The model under review builds one solid part; all positions refer to its coordinate system, in mm. A direction names the side the tool comes from. Round coordinates to 2 decimals unless told otherwise and drop trailing zeros. Write each loop counter-clockwise with the first axis right and the second up, starting at its lowest first coordinate (ties: lowest second). Pieces come first, ordered by that corner, then holes.
Item 1: Draft analysis for pull direction X (two halves, no side actions). For faces 1 (the face through (5.86, 20.83, 6.6)), 2 (the face through (236.99, 31.15, 0.49)), 3 (the face through (118.226, 4.257, 1.521)), 4 (the face through (118, 17, 0)), state which applies: +X half, -X half, draft (parallel to the pull), parting line (faces both ways), or undercut.
Item 2: Machinability: for faces 5 (the face through (118, 8, 4)), 6 (the face through (118, 17, 4)), 7 (the face through (5.86, 16.93, 3.17)), 8 (the face through (234.14, 13.17, 6.72)), 9 (the face through (118, 26, 4)), which of the approach directions +Z, -Z, +X, -X, +Y, -Y give a long, thin tool a straight path to every point of the face, cutting with its end or side? Answer none if there is none.
Item 3: To check wall thickness, follow L1, parallel to Y at x = 26, z = 7; L2, parallel to X at y = 27, z = 2.75; L3, parallel to Y at x = 120, z = 1.7. State the ranges of each line that lie inside material, in increasing order.
Item 4: Clearance check with flat-ended pins moving along their axes: pin 1 Ø3.5 at (x, y) = (124, 6.5) entering from +Z; pin 2 Ø2 at (y, z) = (9.5, 1.5) entering from +X; pin 3 Ø3.5 at (x, z) = (101.5, 9) entering from -Y; pin 4 Ø3 at (x, z) = (70, 8.5) entering from +Y. State where each tip first meets the part, or that it passes through.
Item 5: Add section A-A (z = 8.25). Give the boundary of the cut face in (x, y), plus the area to 3 significant figures.
Item 6: Add section B-B (x = 60). Give the boundary of the cut face in (y, z).
```python
from build123d import *

# Parameters (mm, degrees)
PAD_DEPTH       = 240
FILLET_R        = 10
FILLET001_R     = 3
CHAMFER_1_SIZE2 = 10
CHAMFER_1_SIZE  = 2
CHAMFER_2_SIZE2 = 10
CHAMFER_2_SIZE  = 2
FILLET002_R     = 2
SKETCH001_R     = 2
POCKET_DEPTH    = 4.001
CHAMFER001_SIZE = 1


with BuildPart() as part:
    # Sketch → Pad (new body)
    with BuildSketch(Plane.YZ):
        Polygon((0, 0), (0, 4), (10, 4), (10, 11), (14, 11), (14, 4), (20, 4), (20, 11), (24, 11), (24, 4), (34, 4), (34, 0), align=None)
    extrude(amount=PAD_DEPTH)

    # Fillet
    fillet_edges = [part.edges().sort_by_distance(p)[0] for p in [
        (240, 0, 2),
        (240, 34, 2),
        (0, 0, 2),
        (0, 34, 2),
    ]]
    fillet(fillet_edges, radius=FILLET_R)

    # Fillet001
    fillet001_edges = [part.edges().sort_by_distance(p)[0] for p in [
        (237.071068, 2.928932, 4),
        (120, 0, 4),
        (2.928932, 2.928932, 4),
        (2.928932, 31.071068, 4),
        (120, 34, 4),
        (237.071068, 31.071068, 4),
    ]]
    fillet(fillet001_edges, radius=FILLET001_R)

    # Chamfer 1
    chamfer_1_edges = [part.edges().sort_by_distance(p)[0] for p in [
        (240, 17, 4),
        (240, 20, 7.5),
        (240, 14, 7.5),
    ]]
    chamfer_1_side = part.faces().sort_by_distance((240, 23.821955, 0.5))[0]
    chamfer(chamfer_1_edges, length=CHAMFER_1_SIZE, length2=CHAMFER_1_SIZE2, reference=chamfer_1_side)

    # Chamfer 2
    chamfer_2_edges = [part.edges().sort_by_distance(p)[0] for p in [
        (0, 17, 4),
        (0, 20, 7.5),
        (0, 14, 7.5),
    ]]
    chamfer_2_side = part.faces().sort_by_distance((0, 23.821955, 0.5))[0]
    chamfer(chamfer_2_edges, length=CHAMFER_2_SIZE, length2=CHAMFER_2_SIZE2, reference=chamfer_2_side)

    # Fillet002
    fillet002_edges = [part.edges().sort_by_distance(p)[0] for p in [
        (240, 12, 6.5),
        (240, 17, 2),
        (240, 22, 6.5),
        (0, 22, 6.5),
        (0, 17, 2),
        (0, 12, 6.5),
    ]]
    fillet(fillet002_edges, radius=FILLET002_R)

    # Sketch001 (on Face29 of Fillet002) → Pocket (cut, through all)
    with BuildSketch(Plane(origin=(0, 0, 4), x_dir=(0, -1, 0), z_dir=(0, 0, 1))):
        with Locations((-28.819804, 12)):
            Circle(SKETCH001_R)
        with Locations((-5.180196, 12)):
            Circle(SKETCH001_R)
        with Locations((-5.180196, 120)):
            Circle(SKETCH001_R)
        with Locations((-28.819804, 120)):
            Circle(SKETCH001_R)
        with Locations((-28.819804, 228)):
            Circle(SKETCH001_R)
        with Locations((-5.180196, 228)):
            Circle(SKETCH001_R)
    extrude(amount=-POCKET_DEPTH, mode=Mode.SUBTRACT)

    # Chamfer001
    chamfer001_edges = [part.edges().sort_by_distance(p)[0] for p in [
        (12, 30.819804, 4),
        (12, 7.180196, 4),
        (120, 7.180196, 4),
        (120, 30.819804, 4),
        (228, 30.819804, 4),
        (228, 7.180196, 4),
    ]]
    chamfer(chamfer001_edges, length=CHAMFER001_SIZE)


solid = part.part
```
Numbers:
1. face 1: -X half
1. face 2: +X half
1. face 3: undercut
1. face 4: draft
2. face 5: +Z, +X, -X, -Y
2. face 6: +Z, +X, -X
2. face 7: +Z, -X
2. face 8: +Z, +X
2. face 9: +Z, +X, -X, +Y
3. L1: y = 10 to 14, 20 to 24
3. L2: x = 1.05 to 11.17, 12.83 to 119.17, 120.83 to 227.17, 228.83 to 238.95
3. L3: y = 0.08 to 3.18, 7.18 to 26.82, 30.82 to 33.92
4. pin 1: stops at z = 4
4. pin 2: stops at x = 240
4. pin 3: stops at y = 10
4. pin 4: stops at y = 24
5. outline: (0, 10) - (240, 10) - (240, 10.36) arc R2 ccw to (238.39, 12.32) - (230, 14) - (10, 14) - (1.61, 12.32) arc R2 ccw to (0, 10.36) - close; (0, 23.64) arc R2 ccw to (1.61, 21.68) - (10, 20) - (230, 20) - (238.39, 21.68) arc R2 ccw to (240, 23.64) - (240, 24) - (0, 24) - close
5. area: 1,880 mm2
6. outline: (0, 0) - (34, 0) - (34, 1) arc R3 ccw to (31, 4) - (24, 4) - (24, 11) - (20, 11) - (20, 4) - (14, 4) - (14, 11) - (10, 11) - (10, 4) - (3, 4) arc R3 ccw to (0, 1) - close
